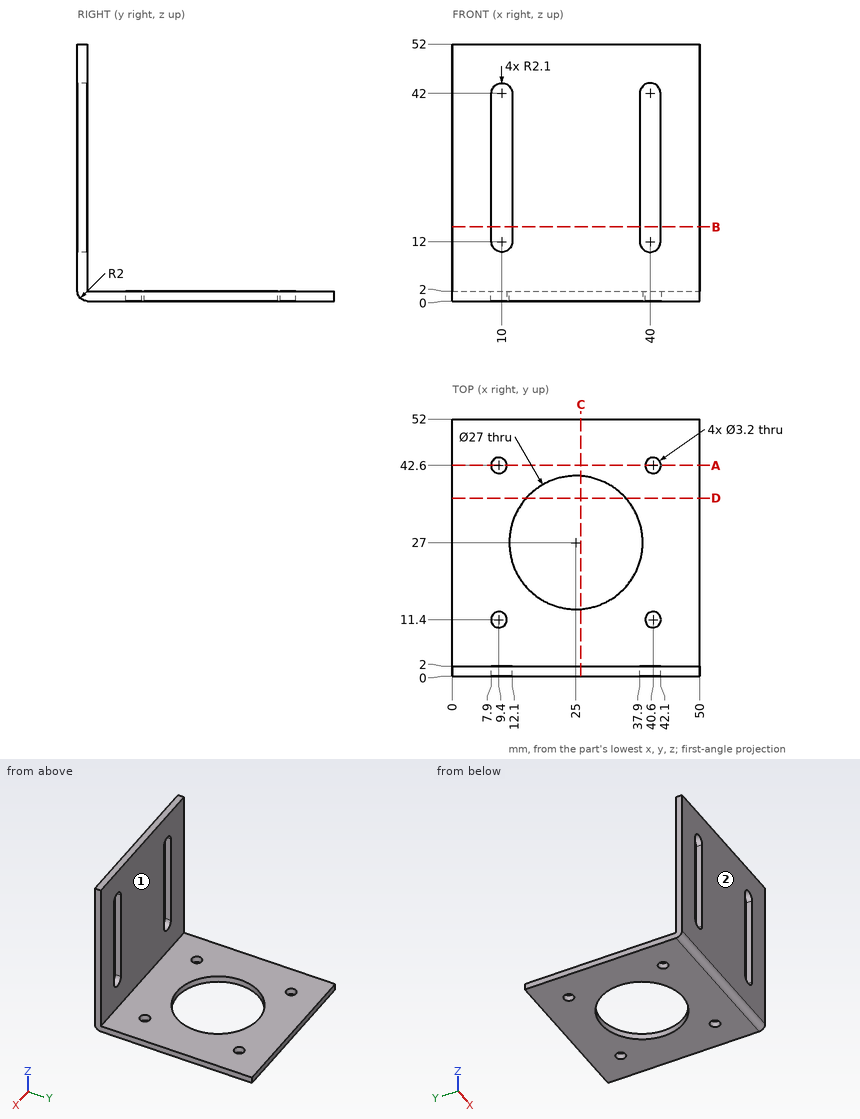
Job drawing, mm, ordinate dimensions from the low corner. One solid piece. A direction names the side the tool comes from. Give positions to 0.01 mm unless a question says otherwise; leave off trailing zeros. Order: outer loops, then holes, each group sorted by start corner. A loop starts at its lowest first (then second) coordinate and runs counter-clockwise, first axis right, second up. Notation, with made-up numbers: (2, 18.5) -> (44, 18.5) arc R14 cw to (44, 32.5) -> close; hole circle Ø11 at (31.25, 18). An arc over 180 degrees is marked (long way). Return JSON: item names as keys, results as strings.
Q1. Saw through at D-D (y = 36). Write the cut outline in (x, z), then the cut area to 3 significant figures.
Working result:
{"outline": "(0, 0) -> (14.94, 0) -> (14.94, 2) -> (0, 2) -> close; (35.06, 0) -> (50, 0) -> (50, 2) -> (35.06, 2) -> close", "area": "59.8 mm²"}
Q2. Drill centre lines: line 1 (Y direction, x = 40.6, z = 1); line 2 (Y direction, x = 30.5, z = 45). Where is each one in solid material? Low to high.
Working result:
{"line 1": "0.27 to 9.8, 13 to 41, 44.2 to 52", "line 2": "0 to 2"}
Q3. Saw through at A-A (y = 42.6). Write the cut outline in (x, z), then the cut area to 3 significant figures.
Working result:
{"outline": "(0, 0) -> (7.8, 0) -> (7.8, 2) -> (0, 2) -> close; (11, 0) -> (39, 0) -> (39, 2) -> (11, 2) -> close; (42.2, 0) -> (50, 0) -> (50, 2) -> (42.2, 2) -> close", "area": "87.2 mm²"}
Q4. Which spindle directions (+Z, -Z, +X, -X, +Y, -Y) get a long thin tool onto all of the face, cutting with end or side? Do the marked faces 1 and 2. Say none if no direction does.
Working result:
{"face 1": "+Z, +X, -X, +Y", "face 2": "+Z, -Z, +X, -X, -Y"}
Q5. Saw through at C-C (x = 26). Write the cut outline in (y, z), then the cut area to 3 significant figures.
Working result:
{"outline": "(0, 2) arc R2 ccw to (2, 0) -> (13.54, 0) -> (13.54, 2) -> (2, 2) -> (2, 52) -> (0, 52) -> close; (40.46, 0) -> (52, 0) -> (52, 2) -> (40.46, 2) -> close", "area": "149 mm²"}
Q6. Saw through at B-B (z = 15). Write the cut outline in (x, y).
Working result:
{"outline": "(0, 0) -> (7.9, 0) -> (7.9, 2) -> (0, 2) -> close; (12.1, 0) -> (37.9, 0) -> (37.9, 2) -> (12.1, 2) -> close; (42.1, 0) -> (50, 0) -> (50, 2) -> (42.1, 2) -> close"}
Q7. Flat gauge pins, fed straight in: pin 1 (12 mm diameter, centred on x = 25, z = 23.5, fed in from +Y); pin 2 (5 mm diameter, centred on x = 9.4, y = 11.4, fed in from +Z). Where does each tip first touch, or does it go through?
Working result:
{"pin 1": "y = 2", "pin 2": "z = 2"}
